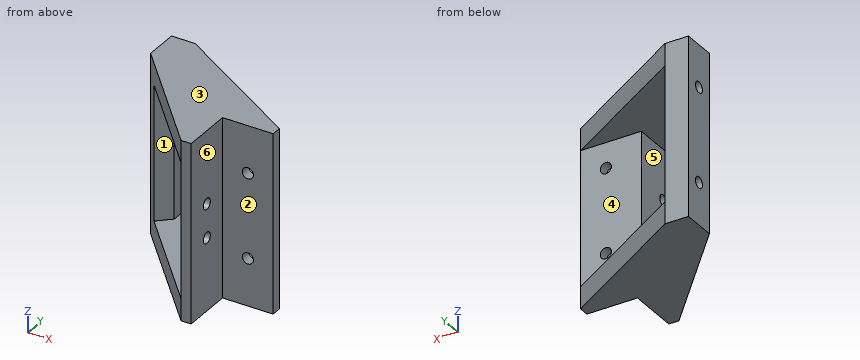
from build123d import *

# Parameters (mm, degrees)
BOSS_EXTRUDE1_DEPTH = 26.5
SKETCH3_W           = 53
SKETCH3_H           = 10
SKETCH3_R           = 1.65
BOSS_EXTRUDE2_DEPTH = 7
CUT_EXTRUDE1_REACH  = 62.402
SKETCH4_W           = 40
SKETCH4_H           = 24.15
CUT_EXTRUDE2_START  = -32.15
SKETCH5_W           = 45
SKETCH5_H           = 40
CUT_EXTRUDE2_DEPTH  = 32.15
SKETCH7_R           = 1.65
CUT_EXTRUDE4_DEPTH  = 3
SKETCH8_R           = 1.65
CUT_EXTRUDE5_DEPTH  = 3
BOSS_EXTRUDE3_REACH = 52.348
SKETCH9_W           = 40
SKETCH9_H           = 4.688556191


with BuildPart() as part:
    # Sketch1 → Boss-Extrude1 (new, symmetric)
    with BuildSketch(Plane.XY):
        Polygon((15, 0), (0, 0), (0, -15), (-3, -15), (-32, 17.15), (-25, 17.15), (-25, 27.15), (15, 3), align=None)
    extrude(amount=BOSS_EXTRUDE1_DEPTH, both=True)

    # Sketch3 → Boss-Extrude2 (add)
    with BuildSketch(Plane.ZY.offset(25)):
        with Locations((0, 22.15)):
            Rectangle(SKETCH3_W, SKETCH3_H)
        with Locations(Location((-14, 22.15, 0), (0, 0, 270))):
            Circle(SKETCH3_R, mode=Mode.SUBTRACT)
        with Locations(Location((14, 22.15, 0), (0, 0, 270))):
            Circle(SKETCH3_R, mode=Mode.SUBTRACT)
    extrude(amount=BOSS_EXTRUDE2_DEPTH)

    # Cut-Extrude1: up to this face of the body (flat: up to its plane)
    cut_extrude1_end = Plane(part.part.faces().sort_by_distance((-25, 22.15, -14))[0])
    # Sketch4 → Cut-Extrude1 (cut, up to the picked face)
    with BuildSketch(Plane(origin=(15, 0, 0), x_dir=(0, 0, -1), z_dir=(1, 0, 0)), mode=Mode.PRIVATE) as cut_extrude1_sk1:
        with Locations((0, 15.075)):
            Rectangle(SKETCH4_W, SKETCH4_H)
    cut_extrude1_tool1 = split(extrude(cut_extrude1_sk1.sketch, amount=-CUT_EXTRUDE1_REACH, mode=Mode.PRIVATE), bisect_by=cut_extrude1_end, keep=Keep.BOTH, mode=Mode.PRIVATE)
    add(cut_extrude1_tool1.solids().sort_by(Axis((15, 15.075, 0), (-1, 0, 0)))[0], mode=Mode.SUBTRACT)

    # Sketch5 → Cut-Extrude2 (cut)
    with BuildSketch(Plane.XZ.offset(15).offset(CUT_EXTRUDE2_START)):
        with Locations((-25.5, 0)):
            Rectangle(SKETCH5_W, SKETCH5_H)
    extrude(amount=CUT_EXTRUDE2_DEPTH, mode=Mode.SUBTRACT)

    # Sketch7 → Cut-Extrude4 (cut)
    with BuildSketch(Plane(origin=(0, 0, 0), x_dir=(0, 0, -1), z_dir=(1, 0, 0))):
        with Locations(Location((-5, -7.5, 0), (0, 0, 90))):
            Circle(SKETCH7_R)
        with Locations(Location((5, -7.5, 0), (0, 0, 90))):
            Circle(SKETCH7_R)
    extrude(amount=-CUT_EXTRUDE4_DEPTH, mode=Mode.SUBTRACT)

    # Sketch8 → Cut-Extrude5 (cut)
    with BuildSketch(Plane.XZ):
        with Locations((7.5, 12.5)):
            Circle(SKETCH8_R)
        with Locations((7.5, -12.5)):
            Circle(SKETCH8_R)
    extrude(amount=-CUT_EXTRUDE5_DEPTH, mode=Mode.SUBTRACT)

    # Boss-Extrude3: up to this face of the body (flat: up to its plane)
    boss_extrude3_end = Plane(part.part.faces().sort_by_distance((-28.5, 17.15, 0))[0])
    # Sketch9 → Boss-Extrude3 (add, up to the picked face)
    with BuildSketch(Plane(origin=(-9.114431039, -8.221415245, 0), x_dir=(0, 0, 1), z_dir=(-0.7425471996920773, -0.669793741557395, 0)), mode=Mode.PRIVATE) as boss_extrude3_sk1:
        with Locations((0, 31.82380611)):
            Rectangle(SKETCH9_W, SKETCH9_H)
    boss_extrude3_tool1 = split(extrude(boss_extrude3_sk1.sketch, amount=-BOSS_EXTRUDE3_REACH, mode=Mode.PRIVATE), bisect_by=boss_extrude3_end, keep=Keep.BOTH, mode=Mode.PRIVATE)
    add(boss_extrude3_tool1.solids().sort_by(Axis((-30.429817, 15.409263, 0), (0.7425471996920773, 0.669793741557395, 0)))[0])


solid = part.part
Work out the finished part from the listing and answer in its coordinate system (mm). Face numbers are marked on the shaded views. A direction names the side the tool comes from. Coordinates: 2 decimals unless noted, no trailing zeros. Write each loop counter-clockwise with the first axis right and the second up, starting at its lowest first coordinate (ties: lowest second). Pieces come first, ordered by that corner, then holes. Notation, with made-up numbers: M 42.25,-17.5 L 81.25,-17.5 A33 ccw 81.25,14.5 Z; hole C 50.25,37 d11. An arc over 180 degrees is marked long. Write item = value, one per line.
1. Flat-ended cylindrical pins translate along their axes: pin 1 (9 mm diameter, centred on x = 10.5, z = -1.5, fed in from +Y); pin 2 (14.5 mm diameter, centred on y = -6, z = 6, fed in from -X); pin 3 (3 mm diameter, centred on x = 7.5, z = -12.5, fed in from +Y); pin 4 (8 mm diameter, centred on y = -4, z = 20, fed in from -X). Find the tip coordinate at first contact, or state that the pin passes through.
Solution:
pin_1 = 3
pin_2 = -3
pin_3 = through
pin_4 = -16.53
2. Straight lines are drawn through the part: line 1 (Z direction, x = 7.5, y = 1.75); line 2 (Z direction, x = -27, y = 22); line 3 (Z direction, x = -23, y = 25). For each, find the intervals that lie inside material, in ascending order. Write a range as from..to.
Solution:
line_1 = -26.5..-14.15, -10.85..10.85, 14.15..26.5
line_2 = -26.5..-15.64, -12.36..12.36, 15.64..26.5
line_3 = -26.5..-20, 20..26.5
3. Determine the mould class of the marked faces 1, 2 and 3 for opening direction Z: released by +Z, released by -Z, zero draft, split by the parting line, or undercut.
Solution:
face_1 = undercut
face_2 = zero draft
face_3 = released by +Z
4. The part is cut by section A-A (z = -19). Determine the outline of the cut face in (x, y).
Solution:
outline = M -32,17.15 L -28.86,13.67 L -25,17.15 L -25,27.15 L -32,27.15 Z; M -3,-15 L 0,-15 L 0,0 L 15,0 L 15,3 L -3,3 Z
5. The part is cut by section C-C (x = -20.5). Determine the outline of the cut face in (y, z).
Solution:
outline = M 4.4,-26.5 L 24.43,-26.5 L 24.43,-20 L 4.4,-20 Z; M 4.4,20 L 24.43,20 L 24.43,26.5 L 4.4,26.5 Z
6. For the marked faces 4, 5 and 6, determine the directions among +Z, -Z, +X, -X, +Y, -Y from which every point of the face is accessible in a straight line to the end or side of a thin tool.
Solution:
face_4 = +X, -X, +Y
face_5 = -X, +Y, -Y
face_6 = +Z, -Z, +X, -Y
7. The part is cut by section B-B (z = -5). Determine the outline of the cut face in (x, y), then the cut area to 3 significant figures.
Solution:
outline = M -32,17.15 L -28.86,13.67 L -25,17.15 L -25,27.15 L -32,27.15 Z; M -3,-15 L 0,-15 L 0,-9.15 L -3,-9.15 Z; M -3,-5.85 L 0,-5.85 L 0,0 L 15,0 L 15,3 L -3,3 Z
area = 171 mm2
8. The part is cut by section D-D (y = 5). Determine the outline of the cut face in (x, z).
Solution:
outline = M -21.04,-26.5 L 11.69,-26.5 L 11.69,-20 L -21.04,-20 Z; M -21.04,20 L 11.69,20 L 11.69,26.5 L -21.04,26.5 Z
